The listing builds one solid part. Answer for the finished solid, in the listing's coordinates (mm). Face numbers are marked on the shaded views. A direction names the side the tool comes from. Round coordinates to 2 decimals unless told otherwise and drop trailing zeros. Loops run counter-clockwise (first coordinate to the right, second up) from the corner with the lowest first, then second, coordinate; pieces in that order, holes last. Notation, with made-up numbers: (-38, 83.5) -> (10, 83.5) arc R11 cw to (10, 95.5) -> close; hole circle Ø10 at (5, -39). An arc over 180 degrees is marked (long way). Use a Markdown table: item, result. Add a question column.
Q1. Given pin 1 Ø2.5 at (y, z) = (16, -7.5) entering from +X; pin 2 Ø5 at (y, z) = (-105, 33.5) entering from -X; pin 3 Ø4 at (x, y) = (0.5, -46) entering from +Z; pin 4 Ø5.5 at (x, z) = (-25, 25) entering from +Y, each flat-ended and moving along its own axis, determine where each tip first touches the part or whether it passes through.
Q2. Section D-D on x = 11 is taken. Give the vertices of the cut face in (y, z).
Q3. For a pull along Z with two mould halves and no side action, classify the marked faces 1, 2, 3 and 4 as released by +Z, released by -Z, zero draft, split by the parting line, or undercut.
Q4. Section C-C on y = -72 is taken. Give the vertices of the cut face in (x, z), then the cut area to 3 significant figures.
Q5. Which of the six approach directions +Z, -Z, +X, -X, +Y, -Y give full straight-line access (tool end or side, diameter ignored) to the marked faces 5, 6, 7 and 8?
Q6. Consider line 1 (X direction, y = -3, z = -25); line 2 (X direction, y = 1.4, z = 0). Determine where each line is inside the solid, lowest interval first.
Q7. Section A-A on z = 0 is taken. Give the vertices of the cut face in (x, y).
from build123d import *

# Parameters (mm, degrees)
SKETCH_2_W               = 60
SKETCH_2_H               = 60
EXTRUDE_1_DEPTH          = 96
SKETCH_3_W               = 10.5
SKETCH_3_H               = 10.5
CUT_EXTRUDE_1_DEPTH      = 97
PATTERN_CIRCULAR_1_COUNT = 4
SKETCH_4_W               = 60
SKETCH_4_H               = 60
EXTRUDE_2_DEPTH          = 6.2
SKETCH_5_R               = 25
EXTRUDE_3_DEPTH          = 3
SKETCH_8_R               = 21.5
SKETCH_8_R_2             = 17.5
CUT_EXTRUDE_3_DEPTH      = 4
SKETCH_9_R               = 15
CUT_EXTRUDE_4_DEPTH      = 3
SKETCH_10_R              = 7
EXTRUDE_5_DEPTH          = 30
FILLET_1_R               = 5
FILLET_2_R               = 2
FILLET_3_R               = 5
SKETCH_13_R              = 28.75
EXTRUDE_6_DEPTH          = 16
EXTRUDE_START            = 16
SKETCH_14_W              = 25
SKETCH_14_H              = 17.123890562
EXTRUDE_7_DEPTH          = 14
EXTRUDE_8_DEPTH          = 2
HOLE_WIZARD_6_0_6_1_D    = 6
CUT_EXTRUDE_5_DEPTH      = 3
EXTRUDE_9_DEPTH          = 5


with BuildPart() as part:
    # Sketch 2 → Extrude 1 (new body)
    with BuildSketch(Plane(origin=(0, 0, 0), x_dir=(1, 0, 0), z_dir=(0, 1, 0))):
        Rectangle(SKETCH_2_W, SKETCH_2_H)
    extrude(amount=-EXTRUDE_1_DEPTH)

    # Sketch 3 → Cut-Extrude 1 (cut, through all)
    with BuildSketch(Plane(origin=(0, 0, 0), x_dir=(1, 0, 0), z_dir=(0, 1, 0))):
        with Locations((-24.75, -24.75)):
            Rectangle(SKETCH_3_W, SKETCH_3_H)
    cut_extrude_1 = extrude(amount=-CUT_EXTRUDE_1_DEPTH, mode=Mode.SUBTRACT)

    # Pattern Circular 1: Cut-Extrude 1 ×4 about axis
    pattern_circular_1_axis = Axis((0, 0, 0), (0, 1, 0))
    for i in range(1, PATTERN_CIRCULAR_1_COUNT):
        add(cut_extrude_1.rotate(pattern_circular_1_axis, i * 360 / PATTERN_CIRCULAR_1_COUNT), mode=Mode.SUBTRACT)

    # Sketch 4 → Extrude 2 (add)
    with BuildSketch(Plane(origin=(0, 0, 0), x_dir=(1, 0, 0), z_dir=(0, 1, 0))):
        Rectangle(SKETCH_4_W, SKETCH_4_H)
    extrude(amount=-EXTRUDE_2_DEPTH)

    # Sketch 5 → Extrude 3 (add)
    with BuildSketch(Plane(origin=(0, 0, 0), x_dir=(1, 0, 0), z_dir=(0, 1, 0))):
        Circle(SKETCH_5_R)
    extrude(amount=EXTRUDE_3_DEPTH)

    # Sketch 8 → Cut-Extrude 3 (cut)
    with BuildSketch(Plane(origin=(0, 3, 0), x_dir=(1, 0, 0), z_dir=(0, 1, 0))):
        Circle(SKETCH_8_R)
        Circle(SKETCH_8_R_2, mode=Mode.SUBTRACT)
    extrude(amount=-CUT_EXTRUDE_3_DEPTH, mode=Mode.SUBTRACT)

    # Sketch 9 → Cut-Extrude 4 (cut)
    with BuildSketch(Plane(origin=(0, 3, 0), x_dir=(1, 0, 0), z_dir=(0, 1, 0))):
        Circle(SKETCH_9_R)
    extrude(amount=-CUT_EXTRUDE_4_DEPTH, mode=Mode.SUBTRACT)

    # Sketch 10 → Extrude 5 (add)
    with BuildSketch(Plane(origin=(0, 0, 0), x_dir=(1, 0, 0), z_dir=(0, 1, 0))):
        Circle(SKETCH_10_R)
    extrude(amount=EXTRUDE_5_DEPTH)

    # Fillet 1
    fillet_1_edges = [part.edges().sort_by_distance(p)[0] for p in [
        (-19.5, -51.1, 19.5),
        (-19.5, -51.1, -19.5),
        (19.5, -51.1, -19.5),
        (19.5, -51.1, 19.5),
    ]]
    fillet(fillet_1_edges, radius=FILLET_1_R)

    # Fillet 2
    fillet_2_edges = [part.edges().sort_by_distance(p)[0] for p in [
        (-30, -51.1, 19.5),
        (-19.5, -51.1, 30),
        (-19.5, -51.1, -30),
        (-30, -51.1, -19.5),
        (30, -51.1, -19.5),
        (19.5, -51.1, -30),
        (19.5, -51.1, 30),
        (30, -51.1, 19.5),
    ]]
    fillet(fillet_2_edges, radius=FILLET_2_R)

    # Fillet 3
    fillet_3_edges = [part.edges().sort_by_distance(p)[0] for p in [
        (30, -3.1, 30),
        (30, -3.1, -30),
        (-30, -3.1, -30),
        (-30, -3.1, 30),
    ]]
    fillet(fillet_3_edges, radius=FILLET_3_R)

    # Sketch 13 → Extrude 6 (add)
    with BuildSketch(Plane.XZ.offset(96)):
        Circle(SKETCH_13_R)
    extrude(amount=EXTRUDE_6_DEPTH)

    # Sketch 14 → Extrude 7 (add)
    with BuildSketch(Plane.XZ.offset(96).offset(EXTRUDE_START)):
        with Locations((7, 29.688054719)):
            Rectangle(SKETCH_14_W, SKETCH_14_H)
    extrude(amount=-EXTRUDE_7_DEPTH)

    # Sketch 15 → Extrude 8 (add)
    with BuildSketch(Plane(origin=(0, -98, 0), x_dir=(1, 0, 0), z_dir=(0, 1, 0))):
        with BuildLine():
            Line((-5.5, -30), (17.5, -30))
            ThreePointArc((17.5, -30), (18.914213562, -29.414213562), (19.5, -28))
            Line((19.5, -28), (19.5, -21.126109438))
            ThreePointArc((19.5, -21.126109438), (7.847121001, -27.658365678), (-5.5, -28.21900955))
            Line((-5.5, -28.21900955), (-5.5, -30))
        make_face()
    extrude(amount=EXTRUDE_8_DEPTH)

    # Hole Wizard 6.0 _6_ _1 (through all)
    with Locations(Plane(origin=(0, 0, 0), x_dir=(1, 0, 0), z_dir=(0, 1, 0))):
        with Locations((-25, 25), (25, 25), (25, -25), (-25, -25)):
            Hole(HOLE_WIZARD_6_0_6_1_D / 2)

    # Sketch 20 → Cut-Extrude 5 (cut)
    with BuildSketch(Plane.XY.offset(-7)):
        with BuildLine():
            Line((-2.5, 24.5), (-2.5, 9.5))
            ThreePointArc((-2.5, 9.5), (0, 7), (2.5, 9.5))
            Line((2.5, 9.5), (2.5, 24.5))
            ThreePointArc((2.5, 24.5), (0, 27), (-2.5, 24.5))
        make_face()
    extrude(amount=CUT_EXTRUDE_5_DEPTH, mode=Mode.SUBTRACT)

    # Sketch 21 → Extrude 9 (add)
    with BuildSketch(Plane(origin=(0, 0, -4), x_dir=(-1, 0, 0), z_dir=(0, 0, -1))):
        with BuildLine():
            Line((2.5, 9.5), (2.5, 24.5))
            ThreePointArc((2.5, 24.5), (0, 27), (-2.5, 24.5))
            Line((-2.5, 24.5), (-2.5, 9.5))
            ThreePointArc((-2.5, 9.5), (0, 7), (2.5, 9.5))
        make_face()
    extrude(amount=EXTRUDE_9_DEPTH)


solid = part.part
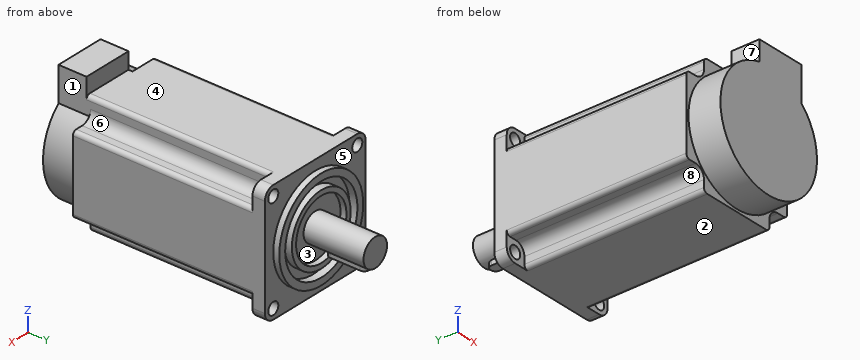
Checked values:
| question | item | result |
|---|---|---|
| 1 | pin 1 | stops at x = 3.15 |
| 1 | pin 2 | stops at x = -5.5 |
| 1 | pin 3 | stops at z = 30 |
| 1 | pin 4 | passes through |
| 2 | outline | (-112, -26.56) -> (-96, -26.56) -> (-96, -30) -> (0, -30) -> (0, -22.45) -> (3, -22.45) -> (3, -18.47) -> (-1, -18.47) -> (-1, -13.61) -> (3, -13.61) -> (3, -10.2) -> (0, -10.2) -> (0, 10.2) -> (3, 10.2) -> (3, 13.61) -> (-1, 13.61) -> (-1, 18.47) -> (3, 18.47) -> (3, 22.45) -> (0, 22.45) -> (0, 30) -> (-98, 30) -> (-98, 38.25) -> (-112, 38.25) -> close |
| 3 | face 1 | zero draft |
| 3 | face 2 | released by -Z |
| 3 | face 3 | undercut |
| 3 | face 4 | released by +Z |
| 4 | outline | (-30, -17.5) arc R2 ccw to (-28, -19.5) -> (-24.5, -19.5) arc R5 cw to (-19.5, -24.5) -> (-19.5, -28) arc R2 ccw to (-17.5, -30) -> (17.5, -30) arc R2 ccw to (19.5, -28) -> (19.5, -24.5) arc R5 cw to (24.5, -19.5) -> (28, -19.5) arc R2 ccw to (30, -17.5) -> (30, 17.5) arc R2 ccw to (28, 19.5) -> (24.5, 19.5) arc R5 cw to (19.5, 24.5) -> (19.5, 28) arc R2 ccw to (17.5, 30) -> (-17.5, 30) arc R2 ccw to (-19.5, 28) -> (-19.5, 24.5) arc R5 cw to (-24.5, 19.5) -> (-28, 19.5) arc R2 ccw to (-30, 17.5) -> close |
| 4 | area | 3,170 mm2 |
| 5 | face 5 | +Y |
| 5 | face 6 | +Z, +X, -Y |
| 5 | face 7 | +Z, -X, -Y |
| 5 | face 8 | -Z, -X, -Y |
| 6 | line 1 | x = -30 to -28, -22 to 22, 28 to 30 |
| 6 | line 2 | x = -25 to -21.5, -17.5 to -15, -7 to 7, 15 to 17.5, 21.5 to 25 |
| 7 | outline | (-30, -96) -> (-28.75, -96) -> (-28.75, -112) -> (28.75, -112) -> (28.75, -96) -> (30, -96) -> (30, 0) -> (25, 0) -> (25, 3) -> (21.5, 3) -> (21.5, -1) -> (17.5, -1) -> (17.5, 3) -> (15, 3) -> (15, 0) -> (7, 0) -> (7, 30) -> (-7, 30) -> (-7, 0) -> (-15, 0) -> (-15, 3) -> (-17.5, 3) -> (-17.5, -1) -> (-21.5, -1) -> (-21.5, 3) -> (-25, 3) -> (-25, 0) -> (-30, 0) -> close |
